Design review of the part built by this model. Coordinates are the model's own, in mm. Coordinates: 2 decimals unless noted, no trailing zeros. Loops run counter-clockwise (first coordinate to the right, second up) from the corner with the lowest first, then second, coordinate; pieces in that order, holes last. Notation, with made-up numbers: M 3.25,76 L 58.25,76 A21 cw 58.25,89 Z; hole C 49.5,21.25 d9. An arc over 180 degrees is marked long. Write item = value, one per line. Start each with the question number.
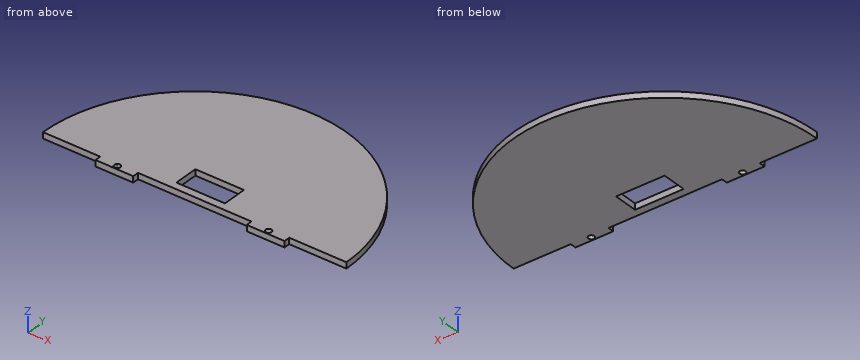
from build123d import *

# Parameters (mm, degrees)
SKETCH1_W           = 25.4
SKETCH1_H           = 12.7
BOSS_EXTRUDE1_DEPTH = 1.59
SKETCH1_4_R         = 1.55
CUT_EXTRUDE2_DEPTH  = 5


with BuildPart() as part:
    # Sketch1 → Boss-Extrude1 (new body, symmetric)
    with BuildSketch(Plane.XY):
        with BuildLine():
            ThreePointArc((79.38, 0), (0, 79.38), (-79.38, 0))
            Line((-79.38, 0), (-49.44, 0))
            Line((-49.44, 0), (-49.44, -3.18))
            Line((-49.44, -3.18), (-29.69, -3.18))
            Line((-29.69, -3.18), (-29.69, 0))
            Line((-29.69, 0), (29.69, 0))
            Line((29.69, 0), (29.69, -3.18))
            Line((29.69, -3.18), (49.44, -3.18))
            Line((49.44, -3.18), (49.44, 0))
            Line((49.44, 0), (79.38, 0))
        make_face()
        with BuildLine():
            ThreePointArc((-40.570037313, 0), (-39.565, 0.37), (-38.559962687, 0))
            Line((-38.559962687, 0), (-40.570037313, 0))
        make_face(mode=Mode.SUBTRACT)
        with Locations((0, 10.35)):
            Rectangle(SKETCH1_W, SKETCH1_H, mode=Mode.SUBTRACT)
    extrude(amount=BOSS_EXTRUDE1_DEPTH, both=True)

    # Sketch1_4 → Cut-Extrude2 (cut, symmetric)
    with BuildSketch(Plane.XY):
        with Locations((-39.565, -1.18)):
            Circle(SKETCH1_4_R)
    cut_extrude2 = extrude(amount=CUT_EXTRUDE2_DEPTH, both=True, mode=Mode.SUBTRACT)

    # Mirror1: Cut-Extrude2 across plane
    add(cut_extrude2.mirror(Plane(origin=(0, 0, 0), x_dir=(0, 0, 1), z_dir=(1, 0, 0))), mode=Mode.SUBTRACT)


solid = part.part
Q1. Add section A-A on x = 0. State the section outline as (y, z) points, plus the area to 3 significant figures.
Q2. Clearance check with flat-ended pins moving along their axes: P1, Ø1, axis at x = 4, z = 0.5, coming from the -Y side; P2, Ø1, axis at x = -2, z = 0, coming from the +Y side; P3, Ø1, axis at y = -1.5, z = -0.5, coming from the -X side. State where each tip first meets the part, or that it passes through.
Q3. Add section B-B on z = 0.95. State the section outline as (x, y) points (3 decimals).
Q4. Add section D-D on x = -66.5. State the section outline as (y, z) points, plus the area to 3 significant figures.
Q5. Add section C-C on y = 60. State the section outline as (x, z) points.
Q6. To check wall thickness, follow line 1 (X direction, y = -1.18, z = -0.35) (3 decimals); line 2 (Y direction, x = -4, z = 0.7); line 3 (Y direction, x = 8, z = -0.25). State the ranges of each line that lie inside material, in increasing order. Write a range as from..to.
Values follow:
q1.outline = M 0,-1.59 L 4,-1.59 L 4,1.59 L 0,1.59 Z; M 16.7,-1.59 L 79.38,-1.59 L 79.38,1.59 L 16.7,1.59 Z
q1.area = 212 mm2
q2.P1 = 0
q2.P2 = 79.37
q2.P3 = -49.44
q3.outline = M -79.38,0 L -49.44,0 L -49.44,-3.18 L -29.69,-3.18 L -29.69,0 L 29.69,0 L 29.69,-3.18 L 49.44,-3.18 L 49.44,0 L 79.38,0 A79.38 ccw Z; hole C -39.565,-1.18 d3.1; hole M -12.7,4 L 12.7,4 L 12.7,16.7 L -12.7,16.7 Z; hole C 39.565,-1.18 d3.1
q4.outline = M 0,-1.59 L 43.35,-1.59 L 43.35,1.59 L 0,1.59 Z
q4.area = 138 mm2
q5.outline = M -51.97,-1.59 L 51.97,-1.59 L 51.97,1.59 L -51.97,1.59 Z
q6.line_1 = -49.44..-41.115, -38.015..-29.69, 29.69..38.015, 41.115..49.44
q6.line_2 = 0..4, 16.7..79.28
q6.line_3 = 0..4, 16.7..78.98
